The drawing under review shows one solid part. Ordinate dimensions are in mm from its lowest x, y, z. A direction names the side the tool comes from. Coordinates: 2 decimals unless noted, no trailing zeros. Order: outer loops, then holes, each group sorted by start corner. A loop starts at its lowest first (then second) coordinate and runs counter-clockwise, first axis right, second up. Notation, with made-up numbers: (-23, 10.25) -> (-6, 10.25) arc R23 ccw to (-6, 47.25) -> close; hole circle Ø9 at (5.5, -35.75). An arc over 180 degrees is marked (long way). Use a Markdown table: item, result. Add a question column.
Q1. Add section C-C (z = 1.2). State the section outline as (x, y) points (1 decimal), then the cut area to 3 significant figures.
Q2. Add section D-D (x = 18). State the section outline as (y, z) points.
Q3. Add section A-A (y = 6). State the section outline as (x, z) points (1 decimal).
Q4. Add section B-B (x = 4). State the section outline as (y, z) points (1 decimal).
Q5. Insertion check: pin 1 (1 mm diameter, centred on y = 22, z = 1, fed in from +X); pin 2 (1 mm diameter, centred on y = 4, z = 1, fed in from -X) (1 decimal); pin 3 (1 mm diameter, centred on x = 18, z = 1, fed in from +Y). Each pin has a flat end and moves straight along its axis. Give the tip position at first contact, or say it passes through.
Q6. The part is to be moulded in two halves that separate along X. For the marked faces 1, 2 and 3, say which applies: pulls with the +X half, pulls with the -X half, needs draft (parallel to the pull), parting line crosses it, or undercut.
Q7. Machinability: for the marked faces 4, 5, 6, 7 and 8, which of the approach directions +Z, -Z, +X, -X, +Y, -Y give a long, thin tool a straight path to every point of the face, cutting with its end or side? Answer none if there is none.
Q8. Wall thickness on probe 1 along Y at (x, z) = (4.25, 0.15) (1 decimal); probe 2 along X at (y, z) = (16.75, 0.5) (1 decimal); probe 3 along Y at (x, z) = (5.5, 1.65) (1 decimal): over which ranges is each line inside the solid? List them lowest first.
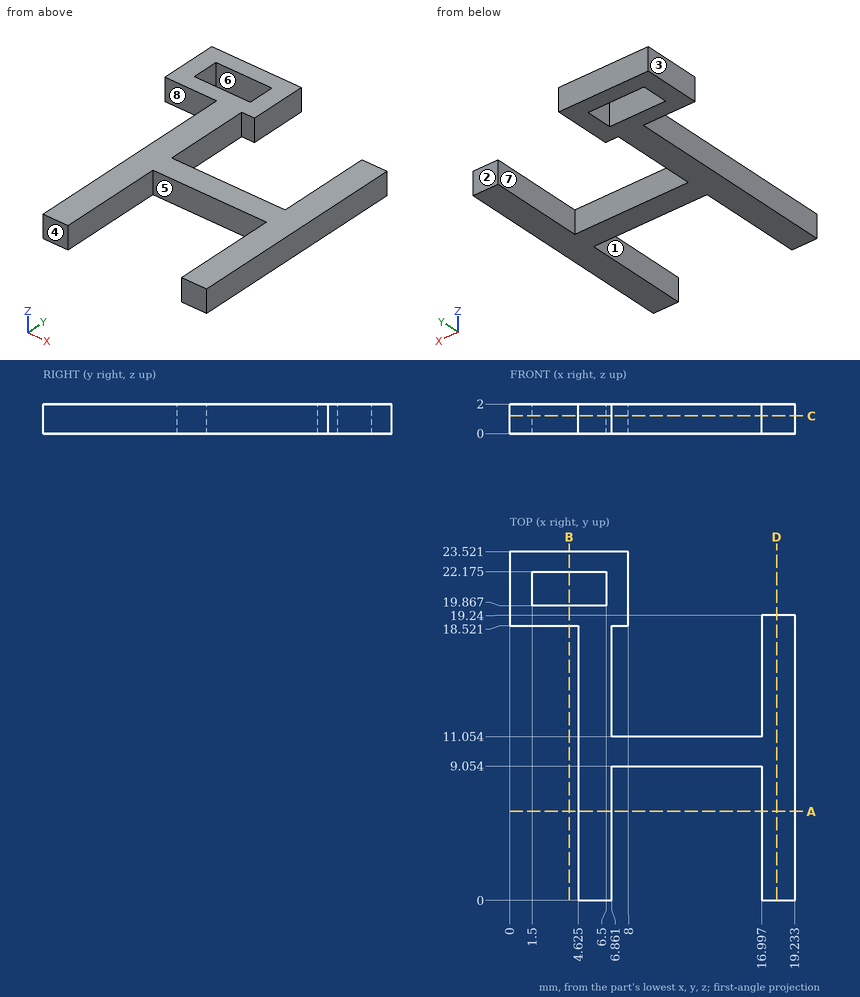
Established:
| question | item | result |
|---|---|---|
| 1 | outline | (0, 18.5) -> (4.6, 18.5) -> (4.6, 0) -> (6.9, 0) -> (6.9, 9.1) -> (17, 9.1) -> (17, 0) -> (19.2, 0) -> (19.2, 19.2) -> (17, 19.2) -> (17, 11.1) -> (6.9, 11.1) -> (6.9, 18.5) -> (8, 18.5) -> (8, 23.5) -> (0, 23.5) -> close; hole (1.5, 19.9) -> (6.5, 19.9) -> (6.5, 22.2) -> (1.5, 22.2) -> close |
| 1 | area | 133 mm^2 |
| 2 | outline | (0, 0) -> (19.24, 0) -> (19.24, 2) -> (0, 2) -> close |
| 3 | outline | (4.6, 0) -> (6.9, 0) -> (6.9, 2) -> (4.6, 2) -> close; (17, 0) -> (19.2, 0) -> (19.2, 2) -> (17, 2) -> close |
| 4 | outline | (18.5, 0) -> (19.9, 0) -> (19.9, 2) -> (18.5, 2) -> close; (22.2, 0) -> (23.5, 0) -> (23.5, 2) -> (22.2, 2) -> close |
| 5 | pin 1 | x = 8 |
| 5 | pin 2 | x = 4.6 |
| 5 | pin 3 | y = 19.24 |
| 6 | face 1 | undercut |
| 6 | face 2 | needs draft |
| 6 | face 3 | pulls with the -X half |
| 7 | face 4 | +Z, -Z, +X, -X, -Y |
| 7 | face 5 | +Z, -Z, -Y |
| 7 | face 6 | +Z, -Z |
| 7 | face 7 | +Z, -Z, +Y |
| 7 | face 8 | +Z, -Z, -X, -Y |
| 8 | probe 1 | 18.5 to 19.9, 22.2 to 23.5 |
| 8 | probe 2 | 4.6 to 6.9, 17 to 19.2 |
| 8 | probe 3 | 0 to 19.9, 22.2 to 23.5 |
